Can you work these out from the model? Positions are in its coordinate system, mm. A direction names the side the tool comes from. Round coordinates to 2 decimals unless told otherwise and drop trailing zeros. Order: outer loops, then holes, each group sorted by start corner. A loop starts at its lowest first (then second) coordinate and runs counter-clockwise, first axis right, second up. Notation, with made-up numbers: (21.5, 12) -> (44.5, 12) arc R22 ccw to (44.5, 51) -> close; hole circle Ø4 at (32, 14). An arc over 180 degrees is marked (long way). One line per item, written item: value.
```python
from build123d import *
from build123d.topology import SkipClean

# Parameters (mm, degrees)
EXTRUDE_1_DEPTH          = 2.5
CUT_EXTRUDE_3_DEPTH      = 26.294674154
CUT_EXTRUDE_3_DEPTH_BACK = 26.294674154
SKETCH_1_3_R             = 2
FILLET_1_R               = 3
EXTRUDE_START            = -1.5
EXTRUDE_2_DEPTH          = 1.5
EXTRUDE_5_DEPTH          = 2.5
SKETCH_2_R               = 1.8
EXTRUDE_4_DEPTH          = 5
SKETCH_3_R               = 0.25
CUT_EXTRUDE_4_DEPTH      = 2


with BuildPart() as part:
    # 草图1 → 凸台-拉伸1 (new body)
    with BuildSketch(Plane(origin=(0, 0, 0), x_dir=(0, 0, -1), z_dir=(1, 0, 0))):
        with BuildLine():
            Line((1.479163916, 3.172077255), (-1.479163916, -3.172077255))
            Line((-1.479163916, -3.172077255), (3.19185305, -3.172077255))
            ThreePointArc((3.19185305, -3.172077255), (4.160128527, -1.715613779), (4.5, 0))
            ThreePointArc((4.5, 0), (4.384156276, 1.014482011), (4.042589444, 1.9767323))
            Line((4.042589444, 1.9767323), (1.479163916, 3.172077255))
        make_face()
        with BuildLine():
            Line((1.084261612, -4.36742221), (-1.479163916, -3.172077255))
            Line((-1.479163916, -3.172077255), (-1.479163916, -4.249949895))
            ThreePointArc((-1.479163916, -4.249949895), (-0.206002169, -4.495282317), (1.084261612, -4.36742221))
        make_face()
        with BuildLine():
            Line((3.19185305, -3.172077255), (-1.479163916, -3.172077255))
            Line((-1.479163916, -3.172077255), (1.084261612, -4.36742221))
            ThreePointArc((1.084261612, -4.36742221), (2.220022869, -3.914268573), (3.19185305, -3.172077255))
        make_face()
        with BuildLine():
            Line((-1.479163916, -4.249949895), (-1.479163916, -3.172077255))
            Line((-1.479163916, -3.172077255), (1.479163916, 3.172077255))
            Line((1.479163916, 3.172077255), (4.042589444, 1.9767323))
            ThreePointArc((4.042589444, 1.9767323), (-3.366850219, 2.985685784), (-1.479163916, -4.249949895))
        make_face()
        with BuildLine():
            ThreePointArc((4.5, 0), (4.160128527, -1.715613779), (3.19185305, -3.172077255))
            Line((3.19185305, -3.172077255), (4.520836084, -3.172077255))
            Line((4.520836084, -3.172077255), (4.520836084, -5.969923204))
            Line((4.520836084, -5.969923204), (10.360395407, -8.692954436))
            ThreePointArc((10.360395407, -8.692954436), (9.969385657, -4.648800879), (13.318723239, -2.348799927))
            Line((13.318723239, -2.348799927), (4.042589444, 1.9767323))
            ThreePointArc((4.042589444, 1.9767323), (4.384156276, 1.014482011), (4.5, 0))
        make_face()
        with BuildLine():
            Line((4.520836084, -3.172077255), (3.19185305, -3.172077255))
            ThreePointArc((3.19185305, -3.172077255), (2.220022869, -3.914268573), (1.084261612, -4.36742221))
            Line((1.084261612, -4.36742221), (4.520836084, -5.969923204))
            Line((4.520836084, -5.969923204), (4.520836084, -3.172077255))
        make_face()
        with BuildLine():
            ThreePointArc((1.084261612, -4.36742221), (-0.206002169, -4.495282317), (-1.479163916, -4.249949895))
            Line((-1.479163916, -4.249949895), (-1.479163916, -18))
            Line((-1.479163916, -18), (4.520836084, -18))
            Line((4.520836084, -18), (4.520836084, -5.969923204))
            Line((4.520836084, -5.969923204), (1.084261612, -4.36742221))
        make_face()
        with BuildLine():
            ThreePointArc((17.594616806, -6.339273926), (16.323758221, -3.414930045), (13.318723239, -2.348799927))
            Line((13.318723239, -2.348799927), (15.073780722, -3.167196671))
            Line((15.073780722, -3.167196671), (12.115452889, -9.511351181))
            Line((12.115452889, -9.511351181), (10.360395407, -8.692954436))
            ThreePointArc((10.360395407, -8.692954436), (14.832177795, -10.143014558), (17.594616806, -6.339273926))
        make_face()
        with BuildLine():
            Line((15.073780722, -3.167196671), (13.318723239, -2.348799927))
            ThreePointArc((13.318723239, -2.348799927), (9.969385657, -4.648800879), (10.360395407, -8.692954436))
            Line((10.360395407, -8.692954436), (12.115452889, -9.511351181))
            Line((12.115452889, -9.511351181), (15.073780722, -3.167196671))
        make_face()
    extrude(amount=EXTRUDE_1_DEPTH)

    # 草图1<3> → 切除-拉伸3 (cut, two sides: drawn at the far end of the back side and taken through both)
    with BuildSketch(Plane(origin=(0, 0, 0), x_dir=(0, 0, -1), z_dir=(1, 0, 0)).offset(-CUT_EXTRUDE_3_DEPTH_BACK)):
        Circle(SKETCH_1_3_R)
        with Locations((13.594616806, -6.339273926)):
            Circle(SKETCH_1_3_R)
    extrude(amount=CUT_EXTRUDE_3_DEPTH + CUT_EXTRUDE_3_DEPTH_BACK, mode=Mode.SUBTRACT)

    # 圆角1
    fillet_1_edges = [part.edges().sort_by_distance(p)[0] for p in [
        (1.25, -2.348799927, -13.318723239),
        (1.25, 1.9767323, -4.042589444),
        (1.25, -8.692954436, -10.360395407),
        (1.25, -5.969923204, -4.520836084),
        (1.25, -4.249949895, 1.479163916),
    ]]
    fillet(fillet_1_edges, radius=FILLET_1_R)

    # 草图1<4> → 凸台-拉伸2 (add)
    with SkipClean():  # the faces are left unmerged after this step: merging them gives an invalid solid
        with BuildSketch(Plane(origin=(0, 0, 0), x_dir=(0, 0, -1), z_dir=(1, 0, 0)).offset(EXTRUDE_START)):
            with BuildLine():
                ThreePointArc((17.594616806, -6.339273926), (16.323758221, -3.414930045), (13.318723239, -2.348799927))
                Line((13.318723239, -2.348799927), (15.073780722, -3.167196671))
                Line((15.073780722, -3.167196671), (14.439853329, -4.526658352))
                ThreePointArc((14.439853329, -4.526658352), (15.281399697, -5.264674709), (15.594616806, -6.339273926))
                ThreePointArc((15.594616806, -6.339273926), (14.669216022, -8.026056818), (12.749380282, -8.1518895))
                Line((12.749380282, -8.1518895), (12.115452889, -9.511351181))
                Line((12.115452889, -9.511351181), (10.360395407, -8.692954436))
                ThreePointArc((10.360395407, -8.692954436), (14.832177795, -10.143014558), (17.594616806, -6.339273926))
            make_face()
            with BuildLine():
                Line((15.073780722, -3.167196671), (13.318723239, -2.348799927))
                ThreePointArc((13.318723239, -2.348799927), (9.969385657, -4.648800879), (10.360395407, -8.692954436))
                Line((10.360395407, -8.692954436), (12.115452889, -9.511351181))
                Line((12.115452889, -9.511351181), (12.749380282, -8.1518895))
                ThreePointArc((12.749380282, -8.1518895), (11.782001231, -5.494037403), (14.439853329, -4.526658352))
                Line((14.439853329, -4.526658352), (15.073780722, -3.167196671))
            make_face()
        extrude(amount=EXTRUDE_2_DEPTH)

    # 草图1<5> → 凸台-拉伸5 (add)
    with BuildSketch(Plane(origin=(0, 0, 0), x_dir=(0, 0, -1), z_dir=(1, 0, 0))):
        with BuildLine():
            ThreePointArc((15.594616806, -6.339273926), (15.281399697, -5.264674709), (14.439853329, -4.526658352))
            Line((14.439853329, -4.526658352), (12.749380282, -8.1518895))
            ThreePointArc((12.749380282, -8.1518895), (14.669216022, -8.026056818), (15.594616806, -6.339273926))
        make_face()
        with BuildLine():
            Line((12.749380282, -8.1518895), (14.439853329, -4.526658352))
            ThreePointArc((14.439853329, -4.526658352), (11.782001231, -5.494037403), (12.749380282, -8.1518895))
        make_face()
    extrude(amount=EXTRUDE_5_DEPTH)

    # 草图2 → 凸台-拉伸4 (add)
    with BuildSketch(Plane(origin=(2.5, 0, 0), x_dir=(0, 0, -1), z_dir=(1, 0, 0))):
        with Locations((13.594616806, -6.339273926)):
            Circle(SKETCH_2_R)
    extrude(amount=EXTRUDE_4_DEPTH)

    # 草图3 → 切除-拉伸4 (cut)
    with BuildSketch(Plane(origin=(7.5, 0, 0), x_dir=(0, 0, -1), z_dir=(1, 0, 0))):
        with Locations((13.594616806, -6.339273926)):
            Circle(SKETCH_3_R)
    extrude(amount=-CUT_EXTRUDE_4_DEPTH, mode=Mode.SUBTRACT)

    # 镜向1: part across plane


with BuildPart() as part_1:
    add(part.part)
    add(part.part.mirror(Plane.ZY.offset(1.5)))


solid = part_1.part
```
Q1. I want a section at A-A on z = 0. List the corners of the cut face in (x, y) for me, plus the area to 3 significant figures.
Answers below:
outline: (-5.5, -18) -> (-3, -18) -> (-3, -2) -> (-5.5, -2) -> close; (-5.5, 2) -> (-3, 2) -> (-3, 4.5) -> (-5.5, 4.5) -> close; (0, -18) -> (2.5, -18) -> (2.5, -2) -> (0, -2) -> close; (0, 2) -> (2.5, 2) -> (2.5, 4.5) -> (0, 4.5) -> close
area: 92.5 mm^2
Q2. I want a section at D-D on z = -8.25. List the corners of the cut face in (x, y) for me.
Answers below:
outline: (-5.5, -7.77) -> (-3, -7.77) -> (-3, 0.01) -> (-5.5, 0.01) -> close; (0, -7.77) -> (2.5, -7.77) -> (2.5, 0.01) -> (0, 0.01) -> close
Q3. I want a section at B-B on y = -15. List the corners of the cut face in (x, z) for me, plus the area to 3 significant figures.
Answers below:
outline: (-5.5, -4.52) -> (-3, -4.52) -> (-3, 1.48) -> (-5.5, 1.48) -> close; (0, -4.52) -> (2.5, -4.52) -> (2.5, 1.48) -> (0, 1.48) -> close
area: 30.0 mm^2
Q4. On a 3-axis mill with a long thin cutter (end or side, diameter ignored), from which of +Z, -Z, +X, -X, +Y, -Y can I reach the whole of each face in a straight line? I mean faces 5 (the face through (7.5, -7, -14)), 6 (the face through (-4.27, -8.7, -10.25)), 7 (the face through (-7.965, -7.435, -12.166)). Say none if no direction works.
Answers below:
face 5: +Z, -Z, +X, +Y, -Y
face 6: +X, -X, -Y
face 7: -X
Q5. We'd pull the mould along Z, two halves only. Please class faces 1 (the face through (1, -14, -4.521)), 2 (the face through (1.27, -4.69, 1.79)), 3 (the face through (-3, -6, -14)), 4 (the face through (-3, -4, -2)): released by +Z, released by -Z, zero draft, split by the parting line, or undercut.
Answers below:
face 1: released by -Z
face 2: released by +Z
face 3: undercut
face 4: zero draft
Q6. I want a section at C-C on x = 1.5. List the corners of the cut face in (y, z) for me, plus the area to 3 significant figures.
Answers below:
outline: (-18, -4.52) -> (-10.68, -4.52) arc R3 cw to (-7.96, -8.79) -> (-8.41, -9.76) arc R3 cw to (-9.08, -10.68) arc R4 ccw (long way) to (-2.35, -13.82) arc R3 cw to (-2.07, -12.72) -> (1.59, -4.87) arc R3 cw to (2.59, -3.68) arc R4.5 ccw (long way) to (-3.61, 2.69) arc R3 cw to (-6.02, 1.48) -> (-18, 1.48) -> close; hole circle Ø4 at (0, 0)
area: 239 mm^2
Q7. Will these pins go through, and if not, where does the flat tip stop? pin 1 Ø5 at (y, z) = (-3.5, 0.5) entering from -X; pin 2 Ø2 at (x, y) = (1, -12.5) entering from +Z; pin 3 Ø8 at (x, y) = (0.5, 2) entering from -Z.
Answers below:
pin 1: x = -5.5
pin 2: z = 1.48
pin 3: z = -12.57
Q8. Please list where these lines run through material, in increasing order: line 1 along X through (y, z) = (-0.5, -2.5); line 2 along X through (y, z) = (-5.5, -13.5); line 3 along Y through (x, z) = (-3.8, 0).
Answers below:
line 1: -5.5 to -3, 0 to 2.5
line 2: -10.5 to -3, 0 to 7.5
line 3: -18 to -2, 2 to 4.5
